Geometry check sheet. Reference: the model listing, model coordinates, mm. Face numbers are marked on the shaded views. A direction names the side the tool comes from. Round coordinates to 2 decimals unless told otherwise and drop trailing zeros. Loops run counter-clockwise (first coordinate to the right, second up) from the corner with the lowest first, then second, coordinate; pieces in that order, holes last. Notation, with made-up numbers: M 52,18.5 L 68,18.5 A24 ccw 68,45.5 Z; hole C 37.5,9.25 d3. An arc over 180 degrees is marked long. Use one line per item in the form item = value. Start each with the question number.
1. Go/stop test with flat-tipped pins: pin 1 (3 mm diameter, centred on x = 0, z = 0, fed in from +Y); pin 2 (1.2 mm diameter, centred on x = 0.5, z = 0, fed in from +Y); pin 3 (0.8 mm diameter, centred on x = 0, z = -0.5, fed in from -Y). Record where each tip stops, or that it passes through.
2. Draft check along Y on the marked faces 1, 2, 3 and 4. Enter one of: pulls with the +Y half, pulls with the -Y half, needs draft (parallel to the pull), parting line crosses it, or undercut.
3. Cross-section at B-B (x = 0). Record the boundary of the cut face in (y, z).
4. Cross-section at A-A (y = 18). Record the boundary of the cut face in (x, z), then the cut area to 3 significant figures.
5. Set-up check for the marked faces 5, 6 and 7: record each of +Z, -Z, +X, -X, +Y, -Y from which the full face is reachable in a straight line by a thin tool's end or side.
6. Cross-section at D-D (y = 8.5). Record the boundary of the cut face in (x, z).
7. Material ranges on line 1 (X direction, y = 14.5, z = 0); line 2 (X direction, y = 16.25, z = 0); line 3 (Y direction, x = 2.5, z = -0.75), recorded low to high.
8. Cross-section at C-C (z = 0). Record the boundary of the cut face in (x, y), then the cut area to 3 significant figures.
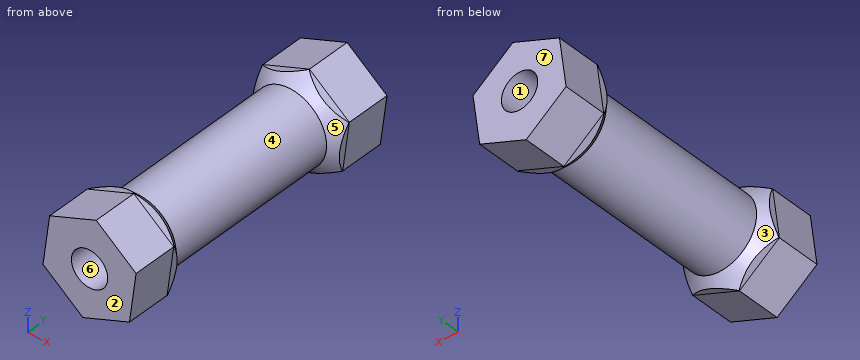
```python
from build123d import *

# Parameters (mm, degrees)
SKETCH_1_R          = 2.5
EXTRUDE_1_DEPTH     = 20
EXTRUDE_2_DEPTH     = 3
EXTRUDE_3_DEPTH     = 3
CHAMFER_1_SIZE      = 1
SKETCH_4_R          = 1.25
CUT_EXTRUDE_1_DEPTH = 8
CUT_EXTRUDE_START   = 8
SKETCH_5_R          = 1.25
CUT_EXTRUDE_2_DEPTH = 8


with BuildPart() as part:
    # 草图1 → 凸台-拉伸1 (new body)
    with BuildSketch(Plane(origin=(0, 0, 0), x_dir=(1, 0, 0), z_dir=(0, 1, 0))):
        with Locations(Location((0, 0, 0), (0, 0, 270))):
            Circle(SKETCH_1_R)
    extrude(amount=EXTRUDE_1_DEPTH)

    # 草图2 → 凸台-拉伸2 (add)
    with BuildSketch(Plane(origin=(0, 20, 0), x_dir=(1, 0, 0), z_dir=(0, 1, 0))):
        Polygon((3.202903935, -1.319623577), (2.744279509, 2.113984385), (-0.458624426, 3.433607962), (-3.202903935, 1.319623577), (-2.744279509, -2.113984385), (0.458624426, -3.433607962), align=None)
    extrude(amount=-EXTRUDE_2_DEPTH)

    # 草图3 → 凸台-拉伸3 (add)
    with BuildSketch(Plane.XZ):
        Polygon((3.202903935, 1.319623577), (0.458624426, 3.433607962), (-2.744279509, 2.113984385), (-3.202903935, -1.319623577), (-0.458624426, -3.433607962), (2.744279509, -2.113984385), align=None)
    extrude(amount=-EXTRUDE_3_DEPTH)

    # 倒角1
    # the kernel refuses this chamfer: 1 mm, written as the material it adds along each edge
    with BuildSketch(Plane(origin=(0, 17, 0), x_dir=(0, 0, 1), z_dir=(1, 0, 0))) as chamfer_1_piece_1_section:
        Polygon((2.5, CHAMFER_1_SIZE), (2.5 + CHAMFER_1_SIZE, 0), (2.5, 0), align=None)
    chamfer_1_piece_1 = revolve(axis=Axis((0, 17, 0), (0, -1, 0)), mode=Mode.PRIVATE)
    chamfer_1_piece_1 = split(chamfer_1_piece_1, bisect_by=Plane(origin=(2.585980682, 16.482096178, -3.299128656), z_dir=(-0.9911972405355005, 0, 0.13239346794615373)), keep=Keep.TOP, mode=Mode.PRIVATE)
    chamfer_1_piece_1 = split(chamfer_1_piece_1, bisect_by=Plane(origin=(3.258731824, 16.482096178, 1.276618014), z_dir=(-0.61025472680424, 0, -0.7922052564917015)), keep=Keep.TOP, mode=Mode.PRIVATE)
    chamfer_1_piece_1 = split(chamfer_1_piece_1, bisect_by=Plane(origin=(0.102470937, 16.482096178, -3.202431915), z_dir=(-0.3809425137312606, 0, 0.924598724437855)), keep=Keep.TOP, mode=Mode.PRIVATE)
    chamfer_1_piece_1 = split(chamfer_1_piece_1, bisect_by=Plane(origin=(-2.183184145, 16.482096178, 2.345160432), z_dir=(0.38094251373126053, 0, -0.924598724437855)), keep=Keep.TOP, mode=Mode.PRIVATE)
    chamfer_1_piece_1 = split(chamfer_1_piece_1, bisect_by=Plane(origin=(-0.402796537, 16.482096178, -3.476613525), z_dir=(0.6102547268042401, 0, 0.7922052564917015)), keep=Keep.TOP, mode=Mode.PRIVATE)
    chamfer_1_piece_1 = split(chamfer_1_piece_1, bisect_by=Plane(origin=(-3.361202761, 16.482096178, -2.504767848), z_dir=(0.9911972405355005, 0, -0.1323934679461537)), keep=Keep.TOP, mode=Mode.PRIVATE)
    add(chamfer_1_piece_1)
    with BuildSketch(Plane(origin=(0, 3, 0), x_dir=(0, 0, 1), z_dir=(1, 0, 0))) as chamfer_1_piece_2_section:
        Polygon((2.5 + CHAMFER_1_SIZE, 0), (2.5, -CHAMFER_1_SIZE), (2.5, 0), align=None)
    chamfer_1_piece_2 = revolve(axis=Axis((0, 3, 0), (0, -1, 0)), mode=Mode.PRIVATE)
    chamfer_1_piece_2 = split(chamfer_1_piece_2, bisect_by=Plane(origin=(3.258731824, 3.517903822, 1.276618014), z_dir=(-0.61025472680424, 0, -0.7922052564917015)), keep=Keep.TOP, mode=Mode.PRIVATE)
    chamfer_1_piece_2 = split(chamfer_1_piece_2, bisect_by=Plane(origin=(2.585980682, 3.517903822, -3.299128656), z_dir=(-0.9911972405355005, 0, 0.13239346794615373)), keep=Keep.TOP, mode=Mode.PRIVATE)
    chamfer_1_piece_2 = split(chamfer_1_piece_2, bisect_by=Plane(origin=(-2.183184145, 3.517903822, 2.345160432), z_dir=(0.38094251373126053, 0, -0.924598724437855)), keep=Keep.TOP, mode=Mode.PRIVATE)
    chamfer_1_piece_2 = split(chamfer_1_piece_2, bisect_by=Plane(origin=(0.102470937, 3.517903822, -3.202431915), z_dir=(-0.3809425137312606, 0, 0.924598724437855)), keep=Keep.TOP, mode=Mode.PRIVATE)
    chamfer_1_piece_2 = split(chamfer_1_piece_2, bisect_by=Plane(origin=(-3.361202761, 3.517903822, -2.504767848), z_dir=(0.9911972405355005, 0, -0.1323934679461537)), keep=Keep.TOP, mode=Mode.PRIVATE)
    chamfer_1_piece_2 = split(chamfer_1_piece_2, bisect_by=Plane(origin=(-0.402796537, 3.517903822, -3.476613525), z_dir=(0.6102547268042401, 0, 0.7922052564917015)), keep=Keep.TOP, mode=Mode.PRIVATE)
    add(chamfer_1_piece_2)

    # 草图4 → 切除-拉伸1 (cut)
    with BuildSketch(Plane(origin=(0, 0, 0), x_dir=(-1, 0, 0), z_dir=(0, 1, 0))):
        with Locations(Location((0, 0, 0), (0, 0, 90))):
            Circle(SKETCH_4_R)
    extrude(amount=CUT_EXTRUDE_1_DEPTH, mode=Mode.SUBTRACT)

    # 草图5 → 切除-拉伸2 (cut)
    with BuildSketch(Plane(origin=(0, 20, 0), x_dir=(-1, 0, 0), z_dir=(0, -1, 0)).offset(CUT_EXTRUDE_START)):
        with Locations(Location((0, 0, 0), (0, 0, 270))):
            Circle(SKETCH_5_R)
    extrude(amount=-CUT_EXTRUDE_2_DEPTH, mode=Mode.SUBTRACT)


solid = part.part
```
Reported:
q1.pin_1 = 20
q1.pin_2 = 12
q1.pin_3 = 8
q2.face_1 = needs draft
q2.face_2 = pulls with the -Y half
q2.face_3 = undercut
q2.face_4 = undercut
q3.outline = M 0,-3.24 L 3.26,-3.24 L 4,-2.5 L 16,-2.5 L 16.74,-3.24 L 20,-3.24 L 20,-1.25 L 12,-1.25 L 12,1.25 L 20,1.25 L 20,3.24 L 16.74,3.24 L 16,2.5 L 4,2.5 L 3.26,3.24 L 0,3.24 L 0,1.25 L 8,1.25 L 8,-1.25 L 0,-1.25 Z
q4.outline = M -3.2,-1.32 L -0.46,-3.43 L 2.74,-2.11 L 3.2,1.32 L 0.46,3.43 L -2.74,2.11 Z; hole C 0,0 d2.5
q4.area = 26.3 mm²
q5.face_5 = none
q5.face_6 = -Y
q5.face_7 = +Z, -Z, +X, -X, +Y
q6.outline = C 0,0 d5
q7.line_1 = -2.5 to -1.25, 1.25 to 2.5
q7.line_2 = -2.75 to -1.25, 1.25 to 2.75
q7.line_3 = 0 to 3.89, 16.11 to 20
q8.outline = M -3.03,0 L -1.25,0 L -1.25,8 L 1.25,8 L 1.25,0 L 3.03,0 L 3.03,3.47 L 2.5,4 L 2.5,16 L 3.03,16.53 L 3.03,20 L 1.25,20 L 1.25,12 L -1.25,12 L -1.25,20 L -3.03,20 L -3.03,16.53 L -2.5,16 L -2.5,4 L -3.03,3.47 Z
q8.area = 67.9 mm²
